Work out the finished part from the listing and answer in its coordinate system (mm). A direction names the side the tool comes from. Give positions to 0.01 mm unless a question says otherwise; leave off trailing zeros. Loops run counter-clockwise (first coordinate to the right, second up) from the corner with the lowest first, then second, coordinate; pieces in that order, holes last. Notation, with made-up numbers: (72, 74) - (86, 74) arc R22 cw to (86, 112) - close; hole circle Ø1 at (37, -39). An arc over 180 degrees is marked (long way). Use CSV: the item, a comma, the result in double quotes.
from build123d import *

# Parameters (mm, degrees)
F0_W           = 20.32
F0_H           = 40.64
F0_R           = 1.016
F0_W_2         = 15.24
F0_H_2         = 31.75
F2_DEPTH       = 17.526
F1_W           = 43.174938
F1_H           = 6.35
F3_DEPTH       = 127
F4_R           = 3.81
F5_DEPTH       = 6.35
F7_D           = 2.032
F7_CSINK_D     = 3.175
F7_CSINK_ANGLE = 82
F8_D           = 4.064
F8_CSINK_D     = 6.35
F8_CSINK_ANGLE = 82


with BuildPart() as f2:
    # F0 (on Top) → F2 (new body, through all)
    with BuildSketch(Plane.XY):
        with BuildLine():
            Line((6.35, -29.367932), (15.24, -13.97))
            Line((15.24, -13.97), (6.5151, -13.97))
            ThreePointArc((6.5151, -13.97), (5.4991, -14.986), (4.4831, -13.97))
            Line((4.4831, -13.97), (-4.4831, -13.97))
            ThreePointArc((-4.4831, -13.97), (-5.4991, -14.986), (-6.5151, -13.97))
            Line((-6.5151, -13.97), (-15.24, -13.97))
            Line((-15.24, -13.97), (-6.35, -29.367932))
            ThreePointArc((-6.35, -29.367932), (0, -33.034106), (6.35, -29.367932))
        make_face()
        with BuildLine():
            Line((6.5151, -13.97), (15.24, -13.97))
            Line((15.24, -13.97), (15.24, 40.64))
            Line((15.24, 40.64), (0, 40.64))
            Line((0, 40.64), (-15.24, 40.64))
            Line((-15.24, 40.64), (-15.24, -13.97))
            Line((-15.24, -13.97), (-6.5151, -13.97))
            ThreePointArc((-6.5151, -13.97), (-5.4991, -12.954), (-4.4831, -13.97))
            Line((-4.4831, -13.97), (4.4831, -13.97))
            ThreePointArc((4.4831, -13.97), (5.4991, -12.954), (6.5151, -13.97))
        make_face()
        with Locations((0, 10.16)):
            Rectangle(F0_W, F0_H, mode=Mode.SUBTRACT)
        with Locations((-5.4991, 34.036)):
            Circle(F0_R, mode=Mode.SUBTRACT)
        with Locations((5.4991, 34.036)):
            Circle(F0_R, mode=Mode.SUBTRACT)
        with Locations((7.62, 56.515)):
            Rectangle(F0_W_2, F0_H_2)
        with Locations((-7.62, 56.515)):
            Rectangle(F0_W_2, F0_H_2)
    extrude(amount=-F2_DEPTH)

    # F1 (on Right) → F3 (intersect, symmetric)
    with BuildSketch(Plane.YZ):
        Polygon((40.64, -6.35), (40.64, 0), (-21.845814, 0), (-32.838694, -13.100805), (-32.838694, -13.97), (-32.838694, -17.526), (-16.989363, -17.526), (-16.989363, -13.97), (-10.595424, -6.35), align=None)
        with Locations((62.227469, -3.175)):
            Rectangle(F1_W, F1_H)
    extrude(amount=F3_DEPTH, both=True, mode=Mode.INTERSECT)

    # F4 (on face) → F5 (join)
    with BuildSketch(Plane(origin=(0, 0, -17.526), x_dir=(1, 0, 0), z_dir=(0, 0, -1))):
        with Locations((0, 22.86)):
            Circle(F4_R)
    extrude(amount=F5_DEPTH)

    # F7 (through all)
    with Locations(Plane(origin=(0, 0, -23.876), x_dir=(1, 0, 0), z_dir=(0, 0, -1))):
        with Locations((0, 22.86)):
            CounterSinkHole(F7_D / 2, F7_CSINK_D / 2, counter_sink_angle=F7_CSINK_ANGLE)

    # F8 (through all)
    with Locations(Plane.XY):
        with Locations((6.35, 46.99), (-6.35, 46.99), (-6.35, 64.77), (6.35, 64.77)):
            CounterSinkHole(F8_D / 2, F8_CSINK_D / 2, counter_sink_angle=F8_CSINK_ANGLE)


solid = f2.part
Item 1: A cutting plane is placed at B-B on y = 1. Determine the outline of the cut face in (x, z).
Determined:
outline,"(-15.24, -6.35) - (-10.16, -6.35) - (-10.16, 0) - (-15.24, 0) - close; (10.16, -6.35) - (15.24, -6.35) - (15.24, 0) - (10.16, 0) - close"
Item 2: Given P1, Ø5.5, axis at x = -6.35, y = 46.99, coming from the -Z side; P2, Ø1.6, axis at x = -5.5, y = -13.97, coming from the -Z side; P3, Ø3, axis at x = 1, z = -2.5, coming from the -Y side; P4, Ø1.1, axis at x = -5, z = -15.5, coming from the +Y side, each flat-ended and moving along its own axis, determine where each tip first touches the part or whether it passes through.
Determined:
P1,"stops at z = -6.35"
P2,"passes through"
P3,"stops at y = -25.2"
P4,"stops at y = -16.99"
Item 3: For faces 1 (the flat face through (0, -16.989, -16)), 2 (the flat face through (0, -21, -23.876)), 3 (the flat face through (0, 30.48, -3)), determine the directions among +Z, -Z, +X, -X, +Y, -Y from which every point of the face is accessible in a straight line to the end or side of a thin tool.
Determined:
face 1,"-Z, +X, -X, +Y"
face 2,"-Z, +X, -X, +Y, -Y"
face 3,"+Z, -Z"
Item 4: The mould has two halves that part along X. Classify faces 4 (the cylindrical face through (-6.085, 66.785, -3.868)), 5 (the flat face through (0.213, -13.837, -10.213)), 6 (the flat face through (-10.86, -21.56, -8.64)): pulls with the +X half, pulls with the -X half, needs draft (parallel to the pull), parting line crosses it, or undercut.
Determined:
face 4,"undercut"
face 5,"needs draft"
face 6,"pulls with the -X half"
Item 5: A cutting plane is placed at A-A on y = 46.99. Determine the outline of the cut face in (x, z) (3 decimals), and give its area (3 significant figures).
Determined:
outline,"(-15.24, -6.35) - (-8.382, -6.35) - (-8.382, -1.315) - (-9.525, 0) - (-15.24, 0) - close; (-4.318, -6.35) - (4.318, -6.35) - (4.318, -1.315) - (3.175, 0) - (-3.175, 0) - (-4.318, -1.315) - close; (8.382, -6.35) - (15.24, -6.35) - (15.24, 0) - (9.525, 0) - (8.382, -1.315) - close"
area,"139 mm²"
Item 6: A cutting plane is placed at D-D on x = 12.5. Determine the outline of the cut face in (y, z), and give its area (3 significant figures).
Determined:
outline,"(-18.72, -17.53) - (-16.99, -17.53) - (-16.99, -13.97) - (-10.6, -6.35) - (72.39, -6.35) - (72.39, 0) - (-18.72, 0) - close"
area,"622 mm²"
Item 7: A cutting plane is placed at C-C on z = -18.5. Determine the outline of the cut face in (x, y).
Determined:
outline,"circle Ø7.62 at (0, -22.86); hole circle Ø2.03 at (0, -22.86)"
Item 8: Find the intervals of material crossed by line 1 (X direction, y = 64.77, z = -2.55); line 2 (Y direction, x = 0, z = -6.25); line 3 (Y direction, x = -6.35, z = -2.4), in increasing order.
Determined:
line 1,"x = -15.24 to -8.38, -4.32 to 4.32, 8.38 to 15.24"
line 2,"y = -27.09 to -23.88, -21.84 to -10.16, 30.48 to 72.39"
line 3,"y = -23.86 to -14.53, -13.41 to -10.16, 30.48 to 33.48, 34.59 to 44.96, 49.02 to 62.74, 66.8 to 72.39"
